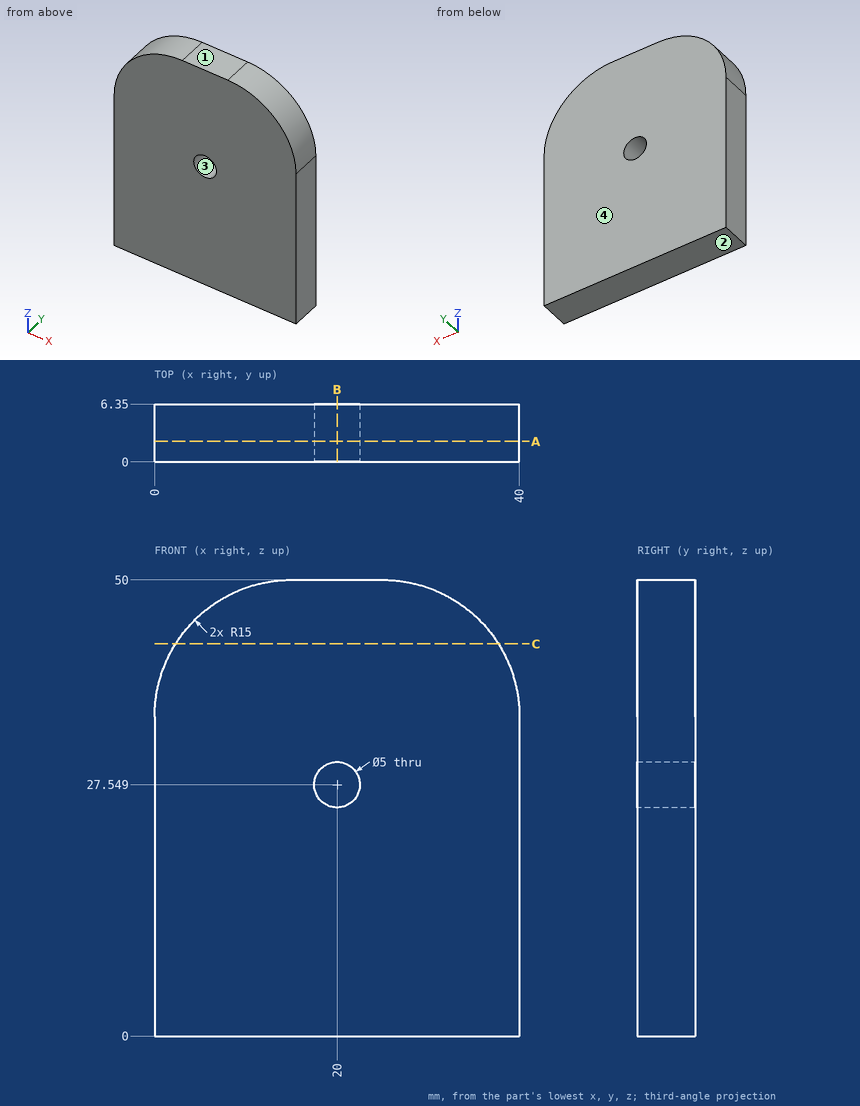
Geometry: see drawing. Coordinates: mm, zero at the bounding-box minimum. Give positions to 0.01 mm unless a question says otherwise; leave off trailing zeros. Write each loop counter-clockwise with the first axis right and the second up, starting at its lowest first coordinate (ties: lowest second). Pieces come first, ordered by that corner, then holes. Notation, with made-up numbers: (-2.5, -8.5) - (14.5, -8.5) arc R14 ccw to (14.5, 8.5) - close; hole circle Ø1 at (-16.5, 18.25). An arc over 180 degrees is marked (long way). Return JSON: item names as keys, results as strings. Group by question number.
1) Section B-B on x = 20. Return the cut outline in (y, z), plus the area to 3 significant figures.
2) First-contact query: P1, Ø1, axis at x = 14, y = 5, coming from the +Z side; P2, Ø1.5, axis at x = 10.5, y = 4, coming from the +Z side; P3, Ø2, axis at y = 1, z = 44, coming from the +X side. Flat tips, straight axial feed; report the tip coordinate or a pass-through.
3) Line query: line 1 (X direction, y = 2.5, z = 28.5); line 2 (X direction, y = 6, z = 28); line 3 (X direction, y = 3, z = 41). Output: solid intervals per line, ascending.
4) Section A-A on y = 2.25. Return the cut outline in (x, z).
5) Mould query, pull axis Z, two halves, no side actions, for the marked faces 1, 2, 3 and 4. Classes: released by +Z, released by -Z, zero draft, split by the parting line, or undercut.
6) Section C-C on z = 43. Return the cut outline in (x, y).
Filled in:
{
 "1": {"outline": "(0, 0) - (6.35, 0) - (6.35, 25.05) - (0, 25.05) - close; (0, 30.05) - (6.35, 30.05) - (6.35, 50) - (0, 50) - close", "area": "286 mm^2"},
 "2": {"P1": "stops at z = 49.99", "P2": "stops at z = 49.52", "P3": "stops at x = 37.69"},
 "3": {"line 1": "x = 0 to 17.69, 22.31 to 40", "line 2": "x = 0 to 17.54, 22.46 to 40", "line 3": "x = 1.25 to 38.75"},
 "4": {"outline": "(0, 0) - (40, 0) - (40, 35) arc R15 ccw to (25, 50) - (15, 50) arc R15 ccw to (0, 35) - close; hole circle Ø5 at (20, 27.55)"},
 "5": {"face 1": "released by +Z", "face 2": "released by -Z", "face 3": "undercut", "face 4": "zero draft"},
 "6": {"outline": "(2.31, 0) - (37.69, 0) - (37.69, 6.35) - (2.31, 6.35) - close"}
}
